The listing builds one solid part. Answer for the finished solid, in the listing's coordinates (mm). Coordinates: 2 decimals unless noted, no trailing zeros. Loops run counter-clockwise (first coordinate to the right, second up) from the corner with the lowest first, then second, coordinate; pieces in that order, holes last. Notation, with made-up numbers: (11, 71) - (51, 71) arc R28 cw to (51, 99) - close; hole circle Ø7 at (80, 38). An arc over 180 degrees is marked (long way). Return JSON: item names as keys, results as strings. Group by question number.
1. Section A-A (z = 1.8) is taken. State how many separate pieces and enclosed holes the cut face has, and give its area (3 significant figures).
2. Find the intervals of material crossed by line 1 along Y through (x, z) = (-125, 1.35); line 2 along Y through (x, z) = (116.5, 1); line 3 along X through (y, z) = (63.5, 2.05), in increasing order.
3. Each of these flat-tipped pins is pushed along its axis until it touches: P1, Ø1, axis at x = -114.5, z = 2, coming from the -Y side; P2, Ø1.5, axis at x = 162, z = 2, coming from the +Y side; P3, Ø1.5, axis at y = -73, z = 2, coming from the -X side. Where does it stop, or does it pass through?
4. Section B-B (x = 176.5) is taken. Write down the section's boundary in (y, z), and give its area (3 significant figures).
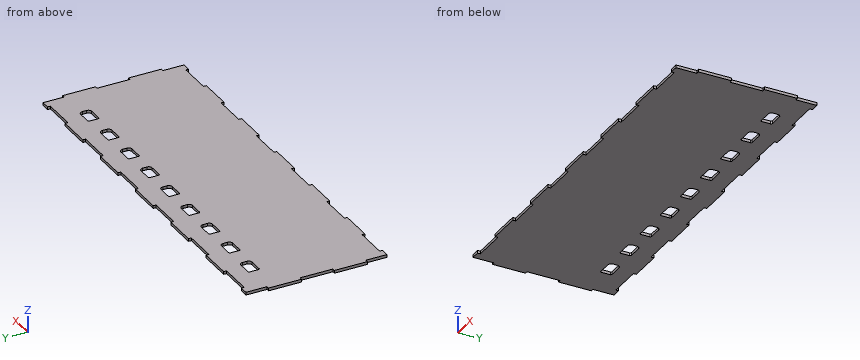
```python
from build123d import *

# Parameters (mm, degrees)
BOSS_EXTRUDE1_DEPTH = 3
CUT_EXTRUDE1_DEPTH  = 218.839964194


with BuildPart() as part:
    # Model → Boss-Extrude1 (new body)
    with BuildSketch(Plane.XY):
        Polygon((201.5, 75), (192.5, 75), (192.5, 72), (157.5, 72), (157.5, 75), (122.5, 75), (122.5, 72), (87.5, 72), (87.5, 75), (52.5, 75), (52.5, 72), (17.5, 72), (17.5, 75), (-17.5, 75), (-17.5, 72), (-52.5, 72), (-52.5, 75), (-87.5, 75), (-87.5, 72), (-122.5, 72), (-122.5, 75), (-157.5, 75), (-157.5, 72), (-192.5, 72), (-192.5, 75), (-201.5, 75), (-201.5, 72), (-201.5, 52.5), (-204.5, 52.5), (-204.5, 17.5), (-201.5, 17.5), (-201.5, -17.5), (-204.5, -17.5), (-204.5, -52.5), (-201.5, -52.5), (-201.5, -72), (-201.5, -75), (-192.5, -75), (-192.5, -72), (-157.5, -72), (-157.5, -75), (-122.5, -75), (-122.5, -72), (-87.5, -72), (-87.5, -75), (-52.5, -75), (-52.5, -72), (-17.5, -72), (-17.5, -75), (17.5, -75), (17.5, -72), (52.5, -72), (52.5, -75), (87.5, -75), (87.5, -72), (122.5, -72), (122.5, -75), (157.5, -75), (157.5, -72), (192.5, -72), (192.5, -75), (201.5, -75), (201.5, -72), (201.5, -52.5), (204.5, -52.5), (204.5, -17.5), (201.5, -17.5), (201.5, 17.5), (204.5, 17.5), (204.5, 52.5), (201.5, 52.5), (201.5, 72), align=None)
    extrude(amount=BOSS_EXTRUDE1_DEPTH)

    # Sketch1 → Cut-Extrude1 (cut, through all)
    with BuildSketch(Plane.XY.offset(3)):
        with BuildLine():
            Line((-154.186662726, 43.1), (-168.461662726, 43.1))
            ThreePointArc((-168.461662726, 43.1), (-169.168769507, 43.392893219), (-169.461662726, 44.1))
            Line((-169.461662726, 44.1), (-169.461662726, 53.8))
            ThreePointArc((-169.461662726, 53.8), (-169.110190863, 54.648528137), (-168.261662726, 55))
            Line((-168.261662726, 55), (-154.386662726, 55))
            ThreePointArc((-154.386662726, 55), (-151.752689966, 53.90897276), (-150.661662726, 51.275))
            Line((-150.661662726, 51.275), (-150.661662726, 46.625))
            ThreePointArc((-150.661662726, 46.625), (-151.694111322, 44.132448596), (-154.186662726, 43.1))
        make_face()
        with BuildLine():
            Line((-114.186662726, 42.283204501), (-128.461662726, 42.283204501))
            ThreePointArc((-128.461662726, 42.283204501), (-129.168769507, 42.57609772), (-129.461662726, 43.283204501))
            Line((-129.461662726, 43.283204501), (-129.461662726, 52.983204501))
            ThreePointArc((-129.461662726, 52.983204501), (-129.110190863, 53.831732638), (-128.261662726, 54.183204501))
            Line((-128.261662726, 54.183204501), (-114.386662726, 54.183204501))
            ThreePointArc((-114.386662726, 54.183204501), (-111.752689966, 53.092177261), (-110.661662726, 50.458204501))
            Line((-110.661662726, 50.458204501), (-110.661662726, 45.808204501))
            ThreePointArc((-110.661662726, 45.808204501), (-111.694111322, 43.315653097), (-114.186662726, 42.283204501))
        make_face()
        with BuildLine():
            Line((-74.186662726, 42.283204501), (-88.461662726, 42.283204501))
            ThreePointArc((-88.461662726, 42.283204501), (-89.168769507, 42.57609772), (-89.461662726, 43.283204501))
            Line((-89.461662726, 43.283204501), (-89.461662726, 52.983204501))
            ThreePointArc((-89.461662726, 52.983204501), (-89.110190863, 53.831732638), (-88.261662726, 54.183204501))
            Line((-88.261662726, 54.183204501), (-74.386662726, 54.183204501))
            ThreePointArc((-74.386662726, 54.183204501), (-71.752689966, 53.092177261), (-70.661662726, 50.458204501))
            Line((-70.661662726, 50.458204501), (-70.661662726, 45.808204501))
            ThreePointArc((-70.661662726, 45.808204501), (-71.694111322, 43.315653097), (-74.186662726, 42.283204501))
        make_face()
        with BuildLine():
            Line((-34.186662726, 42.283204501), (-48.461662726, 42.283204501))
            ThreePointArc((-48.461662726, 42.283204501), (-49.168769507, 42.57609772), (-49.461662726, 43.283204501))
            Line((-49.461662726, 43.283204501), (-49.461662726, 52.983204501))
            ThreePointArc((-49.461662726, 52.983204501), (-49.110190863, 53.831732638), (-48.261662726, 54.183204501))
            Line((-48.261662726, 54.183204501), (-34.386662726, 54.183204501))
            ThreePointArc((-34.386662726, 54.183204501), (-31.752689966, 53.092177261), (-30.661662726, 50.458204501))
            Line((-30.661662726, 50.458204501), (-30.661662726, 45.808204501))
            ThreePointArc((-30.661662726, 45.808204501), (-31.694111322, 43.315653097), (-34.186662726, 42.283204501))
        make_face()
        with BuildLine():
            Line((5.813337274, 42.283204501), (-8.461662726, 42.283204501))
            ThreePointArc((-8.461662726, 42.283204501), (-9.168769507, 42.57609772), (-9.461662726, 43.283204501))
            Line((-9.461662726, 43.283204501), (-9.461662726, 52.983204501))
            ThreePointArc((-9.461662726, 52.983204501), (-9.110190863, 53.831732638), (-8.261662726, 54.183204501))
            Line((-8.261662726, 54.183204501), (5.613337274, 54.183204501))
            ThreePointArc((5.613337274, 54.183204501), (8.247310034, 53.092177261), (9.338337274, 50.458204501))
            Line((9.338337274, 50.458204501), (9.338337274, 45.808204501))
            ThreePointArc((9.338337274, 45.808204501), (8.305888678, 43.315653097), (5.813337274, 42.283204501))
        make_face()
        with BuildLine():
            Line((45.813337274, 42.283204501), (31.538337274, 42.283204501))
            ThreePointArc((31.538337274, 42.283204501), (30.831230493, 42.57609772), (30.538337274, 43.283204501))
            Line((30.538337274, 43.283204501), (30.538337274, 52.983204501))
            ThreePointArc((30.538337274, 52.983204501), (30.889809137, 53.831732638), (31.738337274, 54.183204501))
            Line((31.738337274, 54.183204501), (45.613337274, 54.183204501))
            ThreePointArc((45.613337274, 54.183204501), (48.247310034, 53.092177261), (49.338337274, 50.458204501))
            Line((49.338337274, 50.458204501), (49.338337274, 45.808204501))
            ThreePointArc((49.338337274, 45.808204501), (48.305888678, 43.315653097), (45.813337274, 42.283204501))
        make_face()
        with BuildLine():
            Line((85.813337274, 42.283204501), (71.538337274, 42.283204501))
            ThreePointArc((71.538337274, 42.283204501), (70.831230493, 42.57609772), (70.538337274, 43.283204501))
            Line((70.538337274, 43.283204501), (70.538337274, 52.983204501))
            ThreePointArc((70.538337274, 52.983204501), (70.889809137, 53.831732638), (71.738337274, 54.183204501))
            Line((71.738337274, 54.183204501), (85.613337274, 54.183204501))
            ThreePointArc((85.613337274, 54.183204501), (88.247310034, 53.092177261), (89.338337274, 50.458204501))
            Line((89.338337274, 50.458204501), (89.338337274, 45.808204501))
            ThreePointArc((89.338337274, 45.808204501), (88.305888678, 43.315653097), (85.813337274, 42.283204501))
        make_face()
        with BuildLine():
            Line((125.813337274, 42.283204501), (111.538337274, 42.283204501))
            ThreePointArc((111.538337274, 42.283204501), (110.831230493, 42.57609772), (110.538337274, 43.283204501))
            Line((110.538337274, 43.283204501), (110.538337274, 52.983204501))
            ThreePointArc((110.538337274, 52.983204501), (110.889809137, 53.831732638), (111.738337274, 54.183204501))
            Line((111.738337274, 54.183204501), (125.613337274, 54.183204501))
            ThreePointArc((125.613337274, 54.183204501), (128.247310034, 53.092177261), (129.338337274, 50.458204501))
            Line((129.338337274, 50.458204501), (129.338337274, 45.808204501))
            ThreePointArc((129.338337274, 45.808204501), (128.305888678, 43.315653097), (125.813337274, 42.283204501))
        make_face()
        with BuildLine():
            Line((165.813337274, 42.283204501), (151.538337274, 42.283204501))
            ThreePointArc((151.538337274, 42.283204501), (150.831230493, 42.57609772), (150.538337274, 43.283204501))
            Line((150.538337274, 43.283204501), (150.538337274, 52.983204501))
            ThreePointArc((150.538337274, 52.983204501), (150.889809137, 53.831732638), (151.738337274, 54.183204501))
            Line((151.738337274, 54.183204501), (165.613337274, 54.183204501))
            ThreePointArc((165.613337274, 54.183204501), (168.247310034, 53.092177261), (169.338337274, 50.458204501))
            Line((169.338337274, 50.458204501), (169.338337274, 45.808204501))
            ThreePointArc((169.338337274, 45.808204501), (168.305888678, 43.315653097), (165.813337274, 42.283204501))
        make_face()
    extrude(amount=-CUT_EXTRUDE1_DEPTH, mode=Mode.SUBTRACT)


solid = part.part
```
The answers:
{
 "1": {"separate pieces": "1", "enclosed holes": "9", "area": "57,700 mm2"},
 "2": {"line 1": "y = -75 to 42.28, 54.18 to 75", "line 2": "y = -72 to 42.28, 54.18 to 72", "line 3": "x = -201.5 to 201.5"},
 "3": {"P1": "stops at y = -72", "P2": "stops at y = 72", "P3": "stops at x = -201.5"},
 "4": {"outline": "(-72, 0) - (72, 0) - (72, 3) - (-72, 3) - close", "area": "432 mm2"}
}
